Study the drawing (mm; zero at the part's minimum x, y, z) and answer. A direction names the side the tool comes from. Coordinates: 2 decimals unless noted, no trailing zeros. Loops run counter-clockwise (first coordinate to the right, second up) from the corner with the lowest first, then second, coordinate; pieces in that order, holes last. Notation, with made-up numbers: (-22, 27) - (-1, 27) arc R19 ccw to (-1, 38) - close; hole circle Ø3 at (-11.5, 14.5). An arc over 180 degrees is marked (long way). Use one line per item in the form item = value.
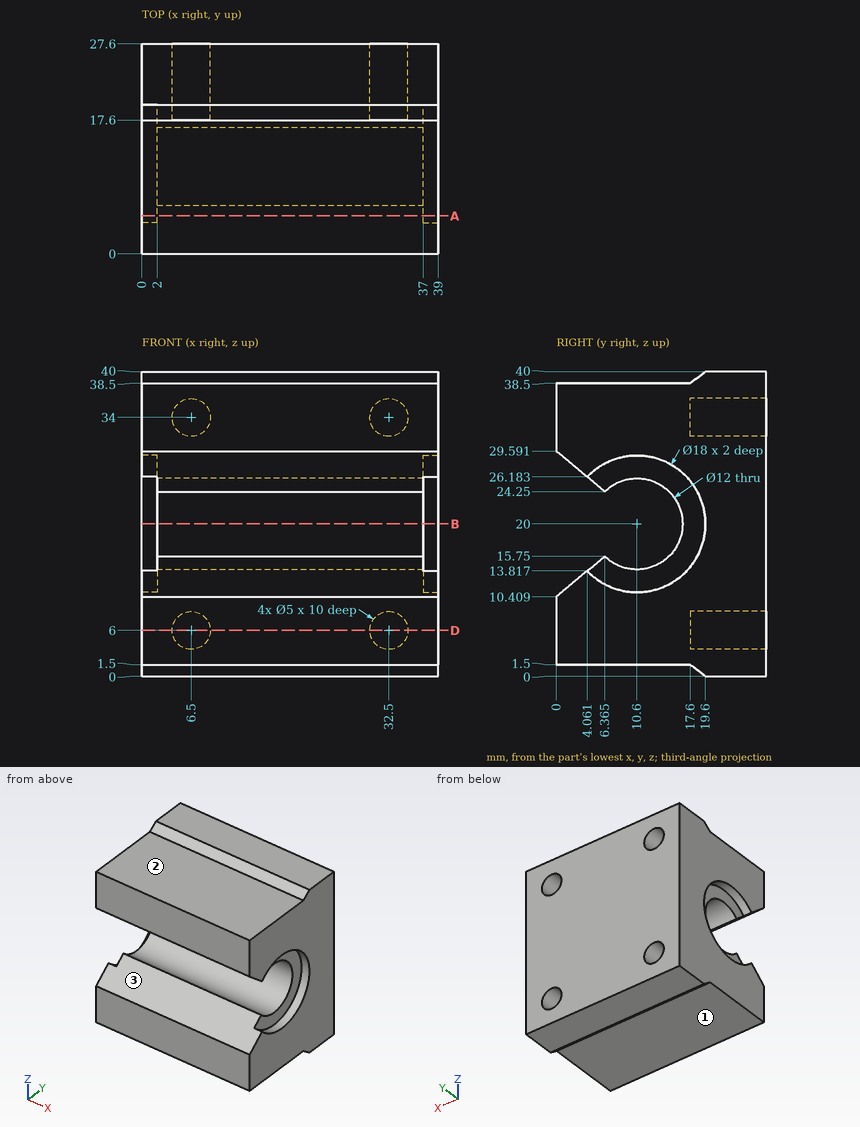
Item 1: The part is cut by section D-D on z = 6. Give the vertices of the cut face in (x, y).
Results below:
outline = (0, 0) - (39, 0) - (39, 27.6) - (35, 27.6) - (35, 17.6) - (30, 17.6) - (30, 27.6) - (9, 27.6) - (9, 17.6) - (4, 17.6) - (4, 27.6) - (0, 27.6) - close
Item 2: The part is cut by section A-A on y = 5. Give the vertices of the cut face in (x, z) (1 decimal), plus the area to 3 significant figures.
Results below:
outline = (0, 1.5) - (39, 1.5) - (39, 13) - (37, 13) - (37, 14.6) - (2, 14.6) - (2, 13) - (0, 13) - close; (0, 27) - (2, 27) - (2, 25.4) - (37, 25.4) - (37, 27) - (39, 27) - (39, 38.5) - (0, 38.5) - close
area = 1,010 mm²
Item 3: Each of these flat-tipped pins is pushed along its axis until it touches: P1, Ø1, axis at y = 6, z = 18, coming from the +X side; P2, Ø9, axis at x = 15, y = 9, coming from the -Z side; P3, Ø2.5, axis at x = 33, z = 7, coming from the +Y side; P4, Ø6, axis at x = 16.5, z = 23.5, coming from the -Y side (1 decimal). Where does it stop, or does it pass through?
Results below:
P1 = through
P2 = 1.5
P3 = 17.6
P4 = 3.7
Item 4: Which of the six approach directions +Z, -Z, +X, -X, +Y, -Y give full straight-line access (tool end or side, diameter ignored) to the marked faces 1, 2 and 3?
Results below:
face_1 = -Z, +X, -X, -Y
face_2 = +Z, +X, -X, -Y
face_3 = +X, -X, -Y
Item 5: Find the intervals of material crossed by L1, parallel to X at y = 25, z = 6; L2, parallel to Z at x = 22.5, y = 17; L3, parallel to X at y = 9.25, z = 28.5, in increasing order.
Results below:
L1 = 0 to 4, 9 to 30, 35 to 39
L2 = 1.5 to 38.5
L3 = 2 to 37
Item 6: The part is cut by section B-B on z = 20. Give the vertices of the cut face in (x, y), plus the area to 3 significant figures.
Results below:
outline = (0, 19.6) - (2, 19.6) - (2, 16.6) - (37, 16.6) - (37, 19.6) - (39, 19.6) - (39, 27.6) - (0, 27.6) - close
area = 417 mm²
